Geometry check sheet. Reference: the model listing, model coordinates, mm. Face numbers are marked on the shaded views. A direction names the side the tool comes from. Coordinates: 2 decimals unless noted, no trailing zeros. Loops run counter-clockwise (first coordinate to the right, second up) from the corner with the lowest first, then second, coordinate; pieces in that order, holes last. Notation, with made-up numbers: M -27.5,29 L 4.5,29 A15 ccw 4.5,52 Z; hole C -26.5,7.25 d11. An arc over 180 degrees is marked long. Use CSV: the item, a comma, the result in double quotes.
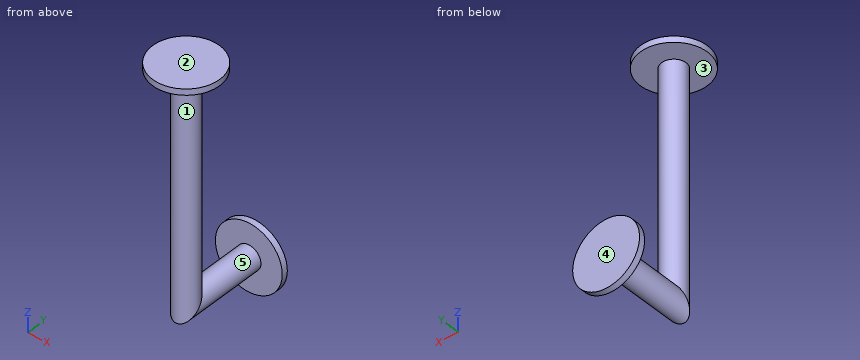
```python
from build123d import *

# Parameters (mm, degrees)
F0_R     = 30
F0_R_2   = 82.5
F3_DEPTH = 15
F4_R     = 82.5
F4_R_2   = 30
F5_DEPTH = 15


with BuildPart() as f2:
    # F2: sweep along a path in F1
    with BuildLine(Plane.YZ) as f2_path:
        Line((0, 0), (-200, 0))
        Line((-200, 0), (-200, 574))
    # F0 (on Front) → F2 (sweep)
    with BuildSketch(Plane.XZ):
        Circle(F0_R)
    sweep(path=f2_path.line, transition=Transition.RIGHT)

    # F0 (on Front) → F3 (join)
    with BuildSketch(Plane.XZ):
        Circle(F0_R_2)
        Circle(F0_R, mode=Mode.SUBTRACT)
    extrude(amount=F3_DEPTH)

    # F4 (on face) → F5 (join)
    with BuildSketch(Plane.XY.offset(574)):
        with Locations((0, -200)):
            Circle(F4_R)
        with Locations((0, -200)):
            Circle(F4_R_2, mode=Mode.SUBTRACT)
    extrude(amount=-F5_DEPTH)


solid = f2.part
```
1. Thickness scan on line 1 (Z direction, x = -64.5, y = -247); line 2 (Y direction, x = 56.5, z = -21); line 3 (Z direction, x = 13.5, y = -118). Record the ranges inside material, lowest first. Write a range as [from, to].
The answers:
line 1,"[559, 574]"
line 2,"[-15, 0]"
line 3,"[-26.79, 26.79]"
2. Section check A-A, the plane y = -200. Record the cut outline in (x, z).
The answers:
outline,"M -82.5,559 L -30,559 L -30,0 A30 ccw 30,0 L 30,559 L 82.5,559 L 82.5,574 L -82.5,574 Z"
3. Section check D-D, the plane z = 50. Record the cut outline in (x, y), plus the area to 3 significant figures.
The answers:
outline,"M -65.62,-15 L 65.62,-15 L 65.62,0 L -65.62,0 Z; C 0,-200 d60"
area,"4,800 mm^2"
4. Section check C-C, the plane x = -68. Record the cut outline in (y, z), plus the area to 3 significant figures.
The answers:
outline,"M -246.71,559 L -153.29,559 L -153.29,574 L -246.71,574 Z; M -15,-46.71 L 0,-46.71 L 0,46.71 L -15,46.71 Z"
area,"2,800 mm^2"
5. Gauge pin test, flat ends, axial feed: P1, Ø12, axis at x = 12, z = 91.5, coming from the -Y side; P2, Ø10, axis at y = -185.5, z = -2, coming from the +X side. Record the tip position at first contact, or that the pin passes through.
The answers:
P1,"y = -229.39"
P2,"x = 30"
6. Section check B-B, the plane x = 0. Record the cut outline in (y, z).
The answers:
outline,"M -282.5,559 L -230,559 L -230,-30 L -15,-30 L -15,-82.5 L 0,-82.5 L 0,82.5 L -15,82.5 L -15,30 L -170,30 L -170,559 L -117.5,559 L -117.5,574 L -282.5,574 Z"
7. Release check for a two-part mould opening along Y. For the marked faces 3, 4 and 5 record: +Y half, -Y half, draft (parallel to the pull), parting line (faces both ways), or undercut.
The answers:
face 3,"draft"
face 4,"+Y half"
face 5,"undercut"
8. Set-up check for the marked faces 1 and 2: record each of +Z, -Z, +X, -X, +Y, -Y from which the full face is reachable in a straight line by a thin tool's end or side.
The answers:
face 1,"none"
face 2,"+Z, +X, -X, +Y, -Y"
